Job drawing, mm, ordinate dimensions from the low corner. One solid piece. A direction names the side the tool comes from. Give positions to 0.01 mm unless a question says otherwise; leave off trailing zeros. Order: outer loops, then holes, each group sorted by start corner. A loop starts at its lowest first (then second) coordinate and runs counter-clockwise, first axis right, second up.
1. Drop flat-ended pins along their axis: pin 1 Ø3 at (y, z) = (49.5, 10) entering from -X; pin 2 Ø12 at (x, z) = (24, 27.5) entering from -Y; pin 3 Ø3 at (x, y) = (24.5, 51) entering from -Z; pin 4 Ø4 at (x, y) = (21, 8) entering from +Z. Give the stop position or say it passes through.
2. Slice it at D-D on y = 8. List the corners of the cut face in (x, z).
3. Slice it at A-A on z = 19. List the corners of the cut face in (x, y), and give its area (3 significant figures).
4. Which spindle directions (+Z, -Z, +X, -X, +Y, -Y) get a long thin tool onto all of the face, cutting with end or side? Do the marked faces 1 and 2. Say none if no direction does.
5. Probe line 1 (Y direction, x = 33.5, z = 8.5); line 2 (Z direction, x = 29, y = 4.5); line 3 (Z direction, x = 13.5, y = 48). List the from-to ranges inside material, lowest first.
6. Slice it at C-C on x = 3. List the corners of the cut face in (y, z).
7. Slice it at B-B on x = 19. List the corners of the cut face in (y, z).
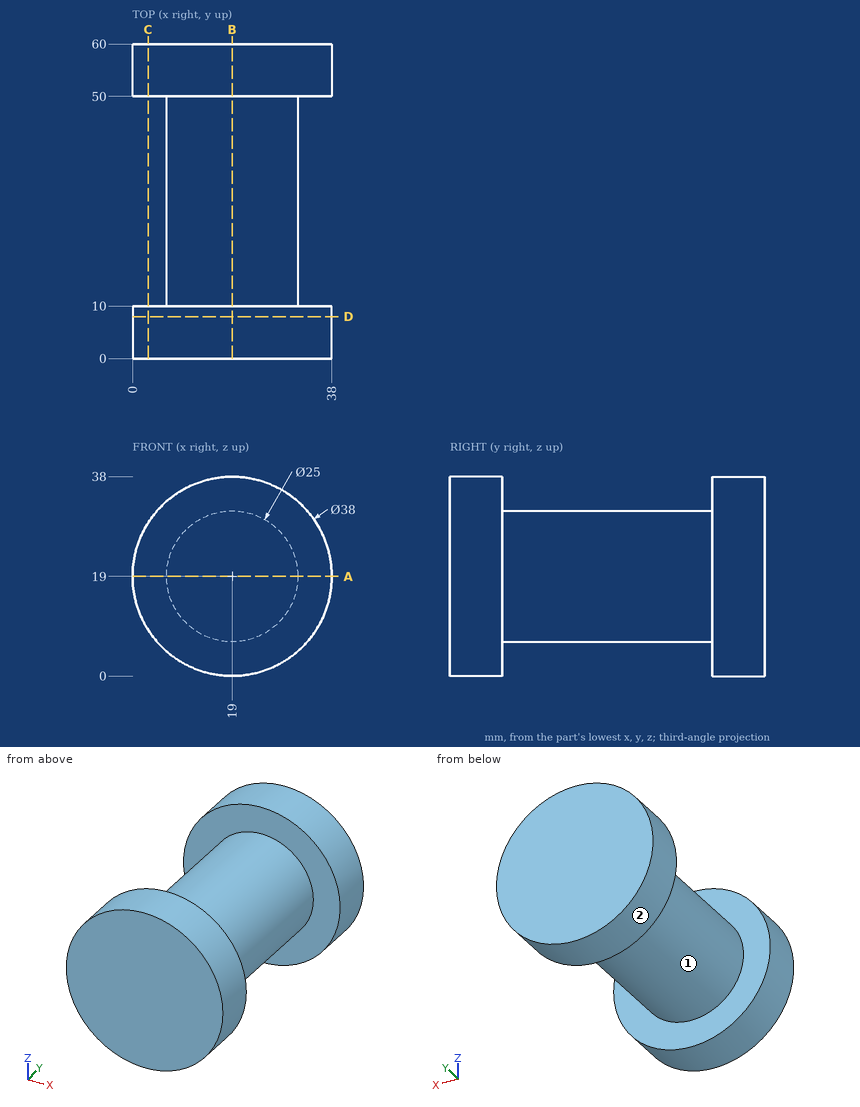
Data:
1. pin 1: stops at x = 1.58
1. pin 2: stops at y = 0
1. pin 3: stops at z = 0.43
1. pin 4: stops at z = 38
2. outline: circle Ø38 at (19, 19)
3. outline: (0, 0) - (38, 0) - (38, 10) - (31.5, 10) - (31.5, 50) - (38, 50) - (38, 60) - (0, 60) - (0, 50) - (6.5, 50) - (6.5, 10) - (0, 10) - close
3. area: 1,760 mm2
4. face 1: none
4. face 2: +Y, -Y
5. line 1: y = 0 to 10, 50 to 60
5. line 2: z = 2.84 to 35.16
5. line 3: z = 7.78 to 30.22
6. outline: (0, 8.75) - (10, 8.75) - (10, 29.25) - (0, 29.25) - close; (50, 8.75) - (60, 8.75) - (60, 29.25) - (50, 29.25) - close
7. outline: (0, 0) - (10, 0) - (10, 6.5) - (50, 6.5) - (50, 0) - (60, 0) - (60, 38) - (50, 38) - (50, 31.5) - (10, 31.5) - (10, 38) - (0, 38) - close
